Check sheet for the modelled part. Datum: model origin and axes. Units: mm. Face numbers are marked on the shaded views. A direction names the side the tool comes from. Round coordinates to 2 decimals unless told otherwise and drop trailing zeros. Order: outer loops, then holes, each group sorted by start corner. A loop starts at its lowest first (then second) coordinate and runs counter-clockwise, first axis right, second up.
Q1. Cross-section at A-A on x = 0. Record the cut outline in (y, z), then the cut area to 3 significant figures.
Q2. Cross-section at B-B on x = 41.5. Record the cut outline in (y, z), then the cut area to 3 significant figures.
Q3. Cross-section at D-D on z = 121. Record the cut outline in (x, y).
Q4. Mould release check, pull along Z, two halves, no side actions. Record for the marked faces 4, 5 and 6: +Z half, -Z half, draft (parallel to the pull), parting line (faces both ways), or undercut.
Q5. Depth check by flat-ended pin: P1, Ø21.5, axis at x = -7.5, y = 6, coming from the -Z side; P2, Ø12, axis at y = 6, z = 115.5, coming from the -X side; P3, Ø1, axis at x = 8, z = 15, coming from the +Y side; P4, Ø21.5, axis at y = -1, z = 79, coming from the +X side. Enter the tip coordinate at first touch or a pass-through.
Q6. Scan lines: probe 1 along Y at (x, z) = (0, 109.95); probe 2 along Z at (x, y) = (30, -10); probe 3 along Z at (x, y) = (-28.5, -23.5). Record each from-to range of solid material in increasing order.
Q7. Cross-section at C-C on y = 40.5. Record the cut outline in (x, z).
Q8. Set-up check for the marked faces 1, 2 and 3: record each of +Z, -Z, +X, -X, +Y, -Y from which the full face is reachable in a straight line by a thin tool's end or side.
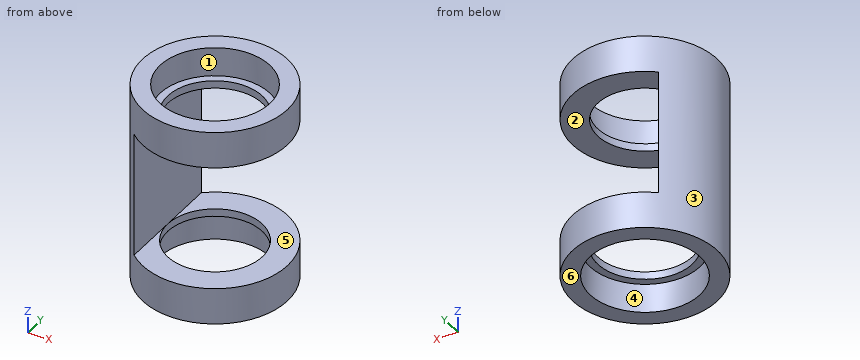
from build123d import *

# Parameters (mm, degrees)
SKETCH_1_R          = 47.5
EXTRUDE_1_DEPTH     = 130
SKETCH_2_R          = 36
CUT_EXTRUDE_1_DEPTH = 19
CUT_EXTRUDE_START   = -19
SKETCH_3_R          = 36
CUT_EXTRUDE_2_DEPTH = 19
SKETCH_4_R          = 31
CUT_EXTRUDE_3_DEPTH = 139
CUT_EXTRUDE_4_DEPTH = 82


with BuildPart() as part:
    # 草图1 → 拉伸1 (new body)
    with BuildSketch(Plane.XY):
        Circle(SKETCH_1_R)
    extrude(amount=EXTRUDE_1_DEPTH)

    # 草图2 → 切除-拉伸1 (cut)
    with BuildSketch(Plane.XY.offset(130)):
        Circle(SKETCH_2_R)
    extrude(amount=-CUT_EXTRUDE_1_DEPTH, mode=Mode.SUBTRACT)

    # 草图3 → 切除-拉伸2 (cut)
    with BuildSketch(Plane(origin=(0, 0, 0), x_dir=(-1, 0, 0), z_dir=(0, 0, -1)).offset(CUT_EXTRUDE_START)):
        with Locations(Location((0, 0, 0), (0, 0, 180))):
            Circle(SKETCH_3_R)
    extrude(amount=CUT_EXTRUDE_2_DEPTH, mode=Mode.SUBTRACT)

    # 草图4 → 切除-拉伸3 (cut)
    with BuildSketch(Plane(origin=(0, 0, 19), x_dir=(-1, 0, 0), z_dir=(0, 0, -1))):
        Circle(SKETCH_4_R)
    extrude(amount=-CUT_EXTRUDE_3_DEPTH, mode=Mode.SUBTRACT)

    # 草图5 → 切除-拉伸4 (cut)
    with BuildSketch(Plane(origin=(0, 0, 24), x_dir=(-1, 0, 0), z_dir=(0, 0, -1))):
        with BuildLine():
            Line((31, -35.989581826), (31, 35.989581826))
            ThreePointArc((31, 35.989581826), (-47.5, 0), (31, -35.989581826))
        make_face()
    extrude(amount=-CUT_EXTRUDE_4_DEPTH, mode=Mode.SUBTRACT)


solid = part.part
Results found:
1. outline: (-47.5, 0) - (-36, 0) - (-36, 19) - (-31, 19) - (-31, 24) - (-47.5, 24) - close; (-47.5, 106) - (-31, 106) - (-31, 111) - (-36, 111) - (-36, 130) - (-47.5, 130) - close; (31, 19) - (36, 19) - (36, 0) - (47.5, 0) - (47.5, 24) - (31, 24) - close; (31, 106) - (47.5, 106) - (47.5, 130) - (36, 130) - (36, 111) - (31, 111) - close
1. area: 1,200 mm2
2. outline: (-23.11, 0) - (23.11, 0) - (23.11, 24) - (-23.11, 24) - close; (-23.11, 106) - (23.11, 106) - (23.11, 130) - (-23.11, 130) - close
2. area: 2,220 mm2
3. outline: circle Ø95 at (0, 0); hole circle Ø72 at (0, 0)
4. face 4: draft
4. face 5: undercut
4. face 6: -Z half
5. P1: passes through
5. P2: stops at x = -47.5
5. P3: stops at y = 46.9
5. P4: stops at x = -31
6. probe 1: y = -47.5 to -31, 31 to 47.5
6. probe 2: z = 19 to 24, 106 to 111
6. probe 3: z = 0 to 24, 106 to 130
7. outline: (-24.82, 0) - (24.82, 0) - (24.82, 24) - (-24.82, 24) - close; (-24.82, 106) - (24.82, 106) - (24.82, 130) - (-24.82, 130) - close
8. face 1: +Z
8. face 2: +X, +Y, -Y
8. face 3: +Z, -Z
